CAD build for the part. Positions are in the model's coordinates, mm. Face numbers are marked on the shaded views. A direction names the side the tool comes from. Coordinates: 2 decimals unless noted, no trailing zeros. Loops run counter-clockwise (first coordinate to the right, second up) from the corner with the lowest first, then second, coordinate; pieces in that order, holes last. Notation, with made-up numbers: (83.25, 82.25) -> (135.25, 82.25) arc R7 cw to (135.25, 93.25) -> close; hole circle Ø10 at (-8, 80). An arc over 180 degrees is marked (long way). Return JSON: item names as keys, results as strings. Group by question number.
(1) Tool access for the marked faces 1 and 2: list every direction of +Z, -Z, +X, -X, +Y, -Y with a clear straight run to the whole face (end or side of a thin tool).
(2) Flat gauge pin, fed straight in: pin 1 Ø1.6 at (x, z) = (8, 1) entering from +Y. Where does the tip first touch, or does it go through?
(3) Mould opens along Z. For the marked faces 3, 4, 5 and 6 say: pulls with the +Z half, pulls with the -Z half, needs draft (parallel to the pull), parting line crosses it, or undercut.
(4) Saw through at A-A on z = 0. Write the cut outline in (x, y).
(5) Saw through at C-C on x = -9.75. Write the cut outline in (y, z).
(6) Probe L1, parallel to X at y = 0.95, z = 0; L2, parallel to X at y = 0.4, z = 1.25; L3, parallel to Z at x = 10, y = 1. List the from-to ranges inside material, lowest first.
(7) Saw through at D-D on z = 2.25. Write the cut outline in (x, y), then the cut area to 3 significant figures.
(8) Saw through at B-B on y = 0.25. Write the cut outline in (x, z), then the cut area to 3 significant figures.
```python
from build123d import *

# Parameters (mm, degrees)
SKETCH1_R           = 2.7305
BOSS_EXTRUDE1_DEPTH = 1.27
BOSS_EXTRUDE2_START = 1.27
BOSS_EXTRUDE2_DEPTH = 1.27


with BuildPart() as part:
    # Sketch1 → Boss-Extrude1 (new body)
    with BuildSketch(Plane(origin=(0, 0, 0), x_dir=(1, 0, 0), z_dir=(0, 1, 0))):
        with BuildLine():
            Line((8.89, -5.08), (-8.89, -5.08))
            ThreePointArc((-8.89, -5.08), (-13.97, 0), (-8.89, 5.08))
            Line((-8.89, 5.08), (8.89, 5.08))
            ThreePointArc((8.89, 5.08), (13.97, 0), (8.89, -5.08))
        make_face()
        with Locations(Location((-8.89, 0, 0), (0, 0, 270))):
            Circle(SKETCH1_R, mode=Mode.SUBTRACT)
        with Locations(Location((8.89, 0, 0), (0, 0, 270))):
            Circle(SKETCH1_R, mode=Mode.SUBTRACT)
    extrude(amount=BOSS_EXTRUDE1_DEPTH)

    # Sketch2 → Boss-Extrude2 (add)
    with BuildSketch(Plane.XZ.offset(BOSS_EXTRUDE2_START)):
        with BuildLine():
            Line((8.89, 5.08), (-8.89, 5.08))
            ThreePointArc((-8.89, 5.08), (-13.97, 0), (-8.89, -5.08))
            Line((-8.89, -5.08), (8.89, -5.08))
            ThreePointArc((8.89, -5.08), (13.97, 0), (8.89, 5.08))
        make_face()
    extrude(amount=-BOSS_EXTRUDE2_DEPTH)


solid = part.part
```
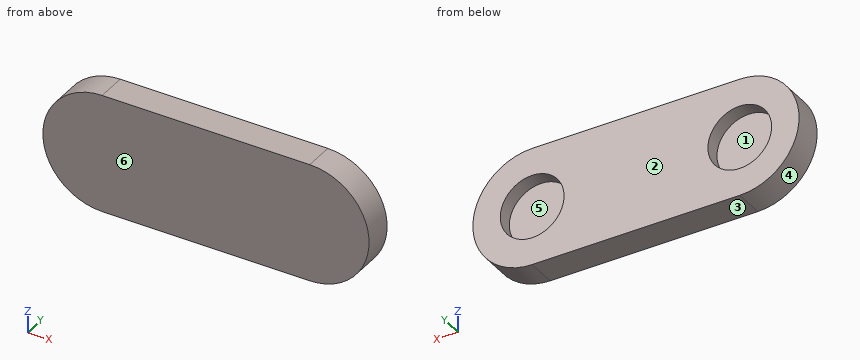
Geometry results:
{
 "1": {"face 1": "+Y", "face 2": "+Z, -Z, +X, -X, +Y"},
 "2": {"pin 1": "y = 0"},
 "3": {"face 3": "pulls with the -Z half", "face 4": "parting line crosses it", "face 5": "undercut", "face 6": "needs draft"},
 "4": {"outline": "(-13.97, -1.27) -> (13.97, -1.27) -> (13.97, 1.27) -> (11.62, 1.27) -> (11.62, 0) -> (6.16, 0) -> (6.16, 1.27) -> (-6.16, 1.27) -> (-6.16, 0) -> (-11.62, 0) -> (-11.62, 1.27) -> (-13.97, 1.27) -> close"},
 "5": {"outline": "(-1.27, -5.01) -> (1.27, -5.01) -> (1.27, -2.59) -> (0, -2.59) -> (0, 2.59) -> (1.27, 2.59) -> (1.27, 5.01) -> (-1.27, 5.01) -> close"},
 "6": {"L1": "-13.97 to -11.62, -6.16 to 6.16, 11.62 to 13.97", "L2": "-13.81 to -11.32, -6.46 to 6.46, 11.32 to 13.81", "L3": "-4.96 to -2.49, 2.49 to 4.96"},
 "7": {"outline": "(-13.44, -1.27) -> (13.44, -1.27) -> (13.44, 1.27) -> (10.44, 1.27) -> (10.44, 0) -> (7.34, 0) -> (7.34, 1.27) -> (-7.34, 1.27) -> (-7.34, 0) -> (-10.44, 0) -> (-10.44, 1.27) -> (-13.44, 1.27) -> close", "area": "60.4 mm²"},
 "8": {"outline": "(-8.89, -5.08) -> (8.89, -5.08) arc R5.08 ccw to (8.89, 5.08) -> (-8.89, 5.08) arc R5.08 ccw to start; hole circle Ø5.46 at (-8.89, 0); hole circle Ø5.46 at (8.89, 0)", "area": "215 mm²"}
}
